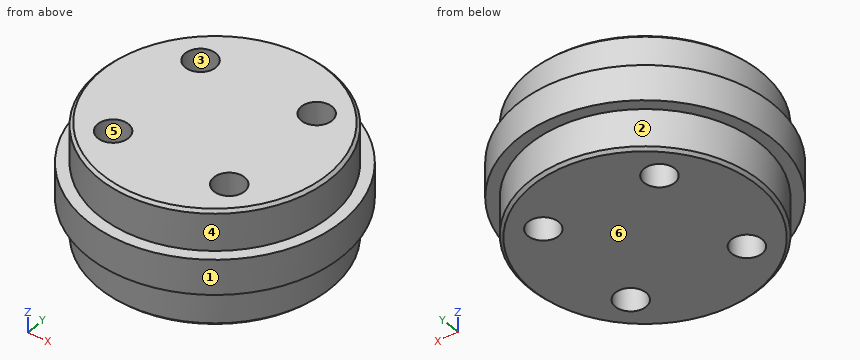
Autodesk Inventor part; units mm, degrees
ref_plane "YZ Plane" through (0, 0, 0) normal (1, 0, 0) x (0, 1, 0)
ref_plane "XZ Plane" through (0, 0, 0) normal (0, 1, 0) x (-1, 0, 0)
ref_plane "XY Plane" through (0, 0, 0) normal (0, 0, 1) x (1, 0, 0)
sketch "スケッチ1" plane through (0, 0, 0) normal (1, 0, 0) x (0, 1, 0)
  line L0 (0, 0) -> (20, 0)
  line L1 (20, -20) -> (0, -20)
  line L2 (0, -20) -> (0, 0)
  line L3 (20, 0) -> (20, -6.95)
  line L4 (20, -6.95) -> (22, -6.95)
  line L5 (22, -6.95) -> (22, -13.05)
  line L6 (22, -13.05) -> (20, -13.05)
  line L7 (20, -13.05) -> (20, -20)
  point P0 (12, 0)
  dimension "d0" = 20
  dimension "d34" = 2
  dimension "d35" = 6.95
  dimension "d36" = 20
  dimension "d37" = 6.95
revolve "回転1" add sketch "スケッチ1" angle 360 about axis through (0, 0, -20) along (0, 0, 1)
chamfer "面取り1" distance 0.5 angle 45 2 edges at (0, -20, 0) (0, -20, -20)
sketch "スケッチ4" plane through (0, 0, -20) normal (0, 0, -1) x (-1, 0, 0)
  line L0 (-10, 10) -> (10, 10)
  line L1 (10, 10) -> (10, -10)
  line L2 (10, -10) -> (-10, -10)
  line L3 (-10, -10) -> (-10, 10)
  line L4 (-10, 10) -> (10, -10) construction
  line L5 (10, 10) -> (-10, -10) construction
  point P0 (0, 0)
  dimension "d24" = 20
  dimension "d25" = 20
hole "穴2" at (-10, 10, -20) at (-10, -10, -20) at (10, -10, -20) at (10, 10, -20) direction (0, 0, 1) diameter 5.3 end through all
ref_plane "作業平面1" through (0, 0, -10) normal (0, 0, 1) x (1, 0, 0)
equation "\"d37\" = d35"
properties part number "scara-base6" material "ABS プラスチック"
Build history of the part. All positions in model axes, mm. Face numbers are marked on the shaded views. A direction names the side the tool comes from. Round coordinates to 2 decimals unless told otherwise and drop trailing zeros. Order: outer loops, then holes, each group sorted by start corner. A loop starts at its lowest first (then second) coordinate and runs counter-clockwise, first axis right, second up. Notation, with made-up numbers: (-2, 66) - (24, 66) arc R22 ccw to (24, 98) - close; hole circle Ø2 at (76, -39.75). An arc over 180 degrees is marked (long way). Use a Markdown table: item, result.
1) Flat gauge pins, fed straight in: pin 1 Ø12 at (y, z) = (-6, -14) entering from -X; pin 2 Ø5 at (x, z) = (5.5, -7) entering from -Y; pin 3 Ø6 at (x, z) = (3.5, -3.5) entering from +Y. Where does each tip first touch, or does it go through?
Recorded:
| item | result |
|---|---|
| pin 1 | stops at x = -22 |
| pin 2 | stops at y = -21.79 |
| pin 3 | stops at y = 19.99 |
2) Saw through at A-A on z = -12. Write the cut outline in (x, y).
Recorded:
| item | result |
|---|---|
| outline | circle Ø44 at (0, 0); hole circle Ø5.3 at (-10, -10); hole circle Ø5.3 at (-10, 10); hole circle Ø5.3 at (10, -10); hole circle Ø5.3 at (10, 10) |
3) Tool access for the marked faces 1 and 2: list every direction of +Z, -Z, +X, -X, +Y, -Y with a clear straight run to the whole face (end or side of a thin tool).
Recorded:
| item | result |
|---|---|
| face 1 | +Z, -Z |
| face 2 | -Z |
4) Pull direction Y, two halves, no side cores. Call the marked faces 3, 4, 5 and 6: pulls with the +Y half, pulls with the -Y half, needs draft (parallel to the pull), parting line crosses it, or undercut.
Recorded:
| item | result |
|---|---|
| face 3 | undercut |
| face 4 | parting line crosses it |
| face 5 | undercut |
| face 6 | needs draft |
5) Saw through at D-D on y = 10. Give the number of separate pieces and of enclosed holes in the cut face, and give its area (3 significant figures).
Recorded:
| item | result |
|---|---|
| separate pieces | 3 |
| enclosed holes | 0 |
| area | 508 mm² |
6) Wall check: L1, parallel to X at y = -10, z = -6; L2, parallel to X at y = -8, z = -11. Give the ranges that are in metal, low to high.
Recorded:
| item | result |
|---|---|
| L1 | x = -17.32 to -12.65, -7.35 to 7.35, 12.65 to 17.32 |
| L2 | x = -20.49 to -11.74, -8.26 to 8.26, 11.74 to 20.49 |
7) Saw through at B-B on y = 0. Write the cut outline in (x, z), and give its area (3 significant figures).
Recorded:
| item | result |
|---|---|
| outline | (-22, -13.05) - (-20, -13.05) - (-20, -19.5) - (-19.5, -20) - (19.5, -20) - (20, -19.5) - (20, -13.05) - (22, -13.05) - (22, -6.95) - (20, -6.95) - (20, -0.5) - (19.5, 0) - (-19.5, 0) - (-20, -0.5) - (-20, -6.95) - (-22, -6.95) - close |
| area | 824 mm² |
